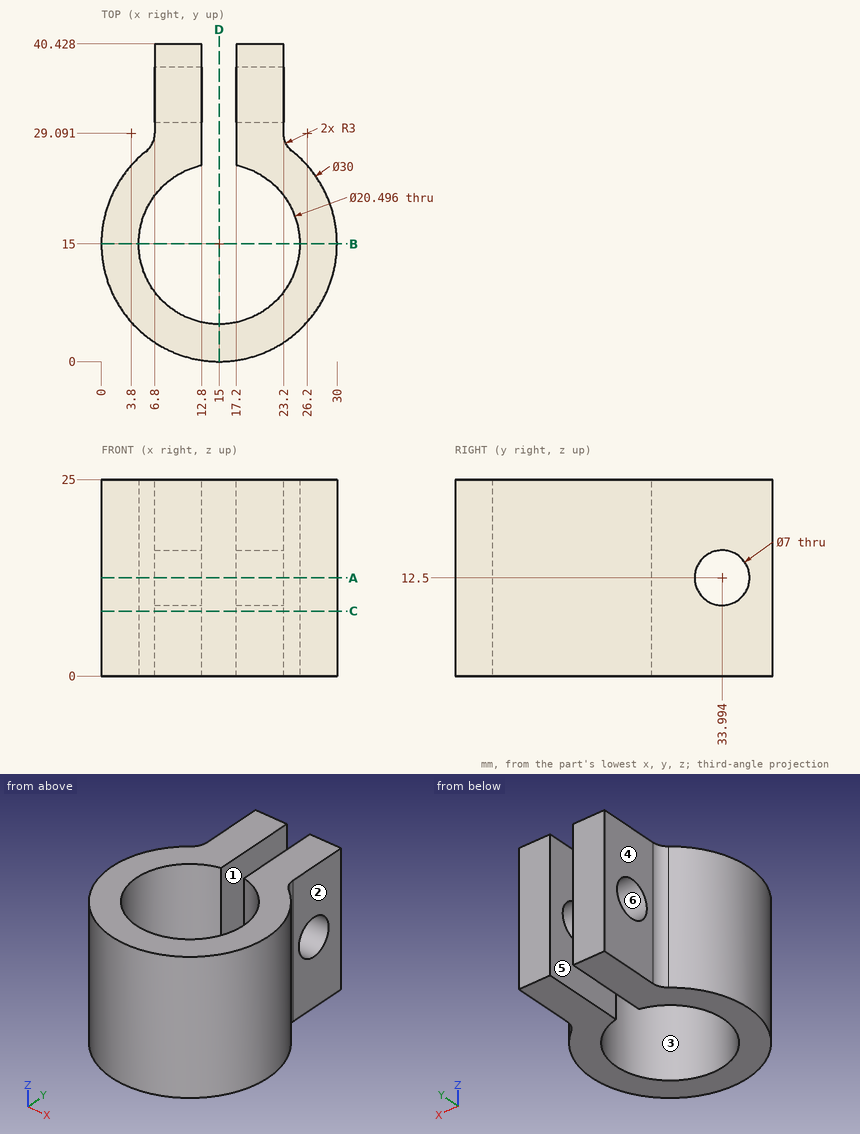
Geometry: see drawing. Coordinates: mm, zero at the bounding-box minimum. A direction names the side the tool comes from. Give positions to 0.01 mm unless a question says otherwise; leave off trailing zeros. Order: outer loops, then holes, each group sorted by start corner. A loop starts at its lowest first (then second) coordinate and runs counter-clockwise, first axis right, second up. Notation, with made-up numbers: (6.25, 59.25) - (19.25, 59.25) arc R32 ccw to (19.25, 95.25) - close; hole circle Ø2 at (65, 57). An arc over 180 degrees is marked (long way). Write each question's results on one line, items separated by ' | '.
Item 1: Section B-B (y = 15). Return loops of the section in (x, z).
A:
outline: (0, 0) - (4.75, 0) - (4.75, 25) - (0, 25) - close; (25.25, 0) - (30, 0) - (30, 25) - (25.25, 25) - close
Item 2: Draft query along X for the marked faces 4, 5 and 6. Return one class per face: released by +X, released by -X, zero draft, split by the parting line, or undercut.
A:
face 4: released by -X | face 5: undercut | face 6: zero draft
Item 3: Section C-C (z = 8.25). Return loops of the section in (x, y).
A:
outline: (5.67, 26.74) arc R15 ccw (long way) to (24.33, 26.74) arc R3 cw to (23.2, 29.09) - (23.2, 40.43) - (17.2, 40.43) - (17.2, 25.01) arc R10.25 cw (long way) to (12.8, 25.01) - (12.8, 40.43) - (6.8, 40.43) - (6.8, 29.09) arc R3 cw to start
Item 4: Contact query for flat-ended pins moving along their axis: pin 1 Ø8 at (y, z) = (33.99, 12.5) entering from -X; pin 2 Ø12 at (x, z) = (5, 11) entering from -Y; pin 3 Ø5 at (x, z) = (5, 15.5) entering from -Y. Output: stop coordinate, or through.
A:
pin 1: stops at x = 6.8 | pin 2: stops at y = 0.54 | pin 3: stops at y = 2.01
Item 5: Section A-A (z = 12.5). Return loops of the section in (x, y).
A:
outline: (5.67, 26.74) arc R15 ccw (long way) to (24.33, 26.74) arc R3 cw to (23.2, 29.09) - (23.2, 30.49) - (17.2, 30.49) - (17.2, 25.01) arc R10.25 cw (long way) to (12.8, 25.01) - (12.8, 30.49) - (6.8, 30.49) - (6.8, 29.09) arc R3 cw to start; (6.8, 37.49) - (12.8, 37.49) - (12.8, 40.43) - (6.8, 40.43) - close; (17.2, 37.49) - (23.2, 37.49) - (23.2, 40.43) - (17.2, 40.43) - close
Item 6: Access query for the marked faces 1, 2 and 3. Directions: +Z, -Z, +X, -X, +Y, -Y. A direction counts if a zero-diameter tool reaches every point of the face in a straight line with its end or side. Return the directions, or none.
A:
face 1: +Z, -Z, +Y | face 2: +Z, -Z, +X, +Y | face 3: +Z, -Z
Item 7: Material intervals for line 1 along Y through (x, z) = (18.5, 9.75) (1 decimal); line 2 along Z through (x, y) = (11.5, 34); line 3 along Y through (x, z) = (18, 12.25) (1 decimal), sorted ascending.
A:
line 1: y = 0.4 to 5.4, 24.6 to 31.8, 36.2 to 40.4 | line 2: z = 0 to 9, 16 to 25 | line 3: y = 0.3 to 5.2, 24.8 to 30.5, 37.5 to 40.4
Item 8: Section D-D (x = 15). Return loops of the section in (y, z).
A:
outline: (0, 0) - (4.75, 0) - (4.75, 25) - (0, 25) - close
